Work out the finished part from the listing and answer in its coordinate system (mm). A direction names the side the tool comes from. Coordinates: 2 decimals unless noted, no trailing zeros. Loops run counter-clockwise (first coordinate to the right, second up) from the corner with the lowest first, then second, coordinate; pieces in that order, holes last.
```python
from build123d import *

# Parameters (mm, degrees)
SKETCH1_R                = 12.7
SKETCH1_R_2              = 10.9
BOSS_EXTRUDE1_DEPTH      = 71
BOSS_EXTRUDE2_DEPTH      = 63
CUT_EXTRUDE1_DEPTH       = 8
CUT_EXTRUDE2_DEPTH       = 15
CUT_EXTRUDE2_DEPTH_BACK  = 16
SKETCH4_R                = 22.297733005
SKETCH5_R                = 2
CUT_EXTRUDE3_DEPTH       = 4
CUT_EXTRUDE4_START       = -4
SKETCH6_R                = 2
CUT_EXTRUDE4_DEPTH       = 4
BOSS_EXTRUDE3_DEPTH      = 6.5
BOSS_EXTRUDE3_DEPTH_BACK = 6.5
SKETCH15_R               = 4
CUT_EXTRUDE14_DEPTH      = 7.5
BOSS_EXTRUDE4_START      = 1.75
SKETCH16_W               = 13
SKETCH16_H               = 13
SKETCH16_R               = 4
BOSS_EXTRUDE4_DEPTH      = 1.75
FILLET1_R                = 2.38
FILLET2_R                = 2.38


with BuildPart() as part:
    # Sketch1 → Boss-Extrude1 (new body)
    with BuildSketch(Plane(origin=(0, 0, 0), x_dir=(1, 0, 0), z_dir=(0, 1, 0))):
        with Locations(Location((0, 0, 0), (0, 0, 270))):
            Circle(SKETCH1_R)
        with Locations(Location((0, 0, 0), (0, 0, 270))):
            Circle(SKETCH1_R_2, mode=Mode.SUBTRACT)
    extrude(amount=BOSS_EXTRUDE1_DEPTH)

    # Sketch2 → Boss-Extrude2 (add)
    with BuildSketch(Plane.XZ):
        with BuildLine():
            Line((12.7, 12.7), (0, 12.7))
            ThreePointArc((0, 12.7), (8.980256121, 8.980256121), (12.7, 0))
            Line((12.7, 0), (12.7, 12.7))
        make_face()
        with BuildLine():
            Line((12.7, -12.7), (12.7, 0))
            ThreePointArc((12.7, 0), (8.980256121, -8.980256121), (0, -12.7))
            Line((0, -12.7), (12.7, -12.7))
        make_face()
    extrude(amount=-BOSS_EXTRUDE2_DEPTH)

    # Sketch3 → Cut-Extrude1 (cut)
    with BuildSketch(Plane.XZ):
        with BuildLine():
            Line((12.7, 12.7), (0, 12.7))
            ThreePointArc((0, 12.7), (8.980256109, 8.980256133), (12.7, 3.4e-08))
            Line((12.7, 3.4e-08), (12.7, 12.7))
        make_face()
        with BuildLine():
            Line((12.7, -12.7), (12.7, 3.4e-08))
            ThreePointArc((12.7, 3.4e-08), (8.980256133, -8.980256109), (0, -12.7))
            Line((0, -12.7), (12.7, -12.7))
        make_face()
    extrude(amount=-CUT_EXTRUDE1_DEPTH, mode=Mode.SUBTRACT)

    # Sketch4 → Cut-Extrude2 (cut, two sides: drawn at the far end of the back side and taken through both)
    with BuildSketch(Plane.XY.offset(-CUT_EXTRUDE2_DEPTH_BACK)):
        with Locations((22.331187996, 35.5)):
            Circle(SKETCH4_R)
    extrude(amount=CUT_EXTRUDE2_DEPTH + CUT_EXTRUDE2_DEPTH_BACK, mode=Mode.SUBTRACT)

    # Sketch5 → Cut-Extrude3 (cut)
    with BuildSketch(Plane(origin=(0, 0, -12.7), x_dir=(-1, 0, 0), z_dir=(0, 0, -1))):
        with Locations((-8.7, 58.5)):
            Circle(SKETCH5_R)
        with Locations((-8.7, 12.5)):
            Circle(SKETCH5_R)
    extrude(amount=-CUT_EXTRUDE3_DEPTH, mode=Mode.SUBTRACT)

    # Sketch6 → Cut-Extrude4 (cut)
    with BuildSketch(Plane.XY.offset(12.7).offset(CUT_EXTRUDE4_START)):
        with Locations(Location((8.7, 58.5, 0), (0, 0, 180))):
            Circle(SKETCH6_R)
        with Locations(Location((8.7, 12.5, 0), (0, 0, 180))):
            Circle(SKETCH6_R)
    extrude(amount=CUT_EXTRUDE4_DEPTH, mode=Mode.SUBTRACT)

    # Sketch14 → Boss-Extrude3 (add, two sides: drawn at the far end of the back side and taken through both)
    with BuildSketch(Plane(origin=(0, 35.5, 0), x_dir=(1, 0, 0), z_dir=(0, 1, 0)).offset(-BOSS_EXTRUDE3_DEPTH_BACK)):
        with BuildLine():
            Line((-14.4365, -6.5), (-14.4365, 6.5))
            Line((-14.4365, 6.5), (-10.836564596, 6.5))
            ThreePointArc((-10.836564596, 6.5), (-12.6365, 0), (-10.836564596, -6.5))
            Line((-10.836564596, -6.5), (-14.4365, -6.5))
        make_face()
    extrude(amount=BOSS_EXTRUDE3_DEPTH + BOSS_EXTRUDE3_DEPTH_BACK)

    # Sketch15 → Cut-Extrude14 (cut)
    with BuildSketch(Plane.ZY.offset(14.4365)):
        with Locations((0, 35.5)):
            Circle(SKETCH15_R)
    extrude(amount=-CUT_EXTRUDE14_DEPTH, mode=Mode.SUBTRACT)

    # Sketch16 → Boss-Extrude4 (add)
    with BuildSketch(Plane.ZY.offset(14.4365).offset(BOSS_EXTRUDE4_START)):
        with Locations((0, 35.5)):
            Rectangle(SKETCH16_W, SKETCH16_H)
        with Locations((0, 35.5)):
            Circle(SKETCH16_R, mode=Mode.SUBTRACT)
    extrude(amount=-BOSS_EXTRUDE4_DEPTH)

    # Fillet1
    fillet1_edges = [part.edges().sort_by_distance(p)[0] for p in [
        (-13.548522679, 29, 6.5),
        (-13.548522679, 29, -6.5),
        (-13.548522679, 42, -6.5),
        (-13.548522679, 42, 6.5),
    ]]
    fillet(fillet1_edges, radius=FILLET1_R)

    # Fillet2
    fillet2_edges = [part.edges().sort_by_distance(p)[0] for p in [
        (12.7, 15.389576958, 0),
        (12.7, 55.610423042, 0),
    ]]
    fillet(fillet2_edges, radius=FILLET2_R)


solid = part.part
```
1. A cutting plane is placed at B-B, the plane x = 5. Give the vertices of the cut face in (y, z).
2. Straight lines are drawn through the part: probe 1 along Y at (x, z) = (8.7, 11.5); probe 2 along X at (y, z) = (58.5, 9.85); probe 3 along Z at (x, y) = (-0.5, 3). For each, find the intervals that lie inside material, in ascending order.
3. A cutting plane is placed at A-A, the plane z = 9.75. Give the vertices of the cut face in (x, y).
4. Each of these flat-tipped pins is pushed along its axis until it touches: P1, Ø1.6, axis at x = -14, y = 36, coming from the +Z side; P2, Ø13, axis at y = 35.5, z = 0, coming from the +X side; P3, Ø4, axis at y = 26, z = -7, coming from the +X side; P4, Ø6.5, axis at x = 4.5, z = -4.5, coming from the -Y side. Where does it stop, or does it pass through?
5. For faces 4 (the cylindrical face through (-13.585, 29.716, -5.821)), 5 (the flat face through (10, 63, -10)), 6 (the cylindrical face through (7.625, 14.186, -10.728)), 7 (the flat face through (9, 12, 8.7)), determine the directions among +Z, -Z, +X, -X, +Y, -Y from which every point of the face is accessible in a straight line to the end or side of a thin tool.
6. A cutting plane is placed at D-D, the plane z = -0.75. Count the separate pieces of the cut face and the enclosed holes in it, then the cut area to 3 significant figures.
7. Determine the mould class of faces 1 (the cylindrical face through (-13.205, 35.676, -3.996)), 2 (the flat face through (0.6, 29, -12.7)), 3 (the flat face through (12.7, 11, 0)) for opening direction Z: released by +Z, released by -Z, zero draft, split by the parting line, or undercut.
8. A cutting plane is placed at C-C, the plane y = 12.5. Give the vertices of the cut face in (x, z), then the cut area to 3 significant figures.
Answers below:
1. outline: (0, -11.67) - (8, -11.67) - (8, -12.7) - (21.47, -12.7) - (21.47, -9.69) - (0, -9.69) - close; (0, 9.69) - (21.47, 9.69) - (21.47, 12.7) - (8, 12.7) - (8, 11.67) - (0, 11.67) - close; (49.53, -12.7) - (63, -12.7) - (63, -11.67) - (71, -11.67) - (71, -9.69) - (49.53, -9.69) - close; (49.53, 9.69) - (71, 9.69) - (71, 11.67) - (63, 11.67) - (63, 12.7) - (49.53, 12.7) - close
2. probe 1: y = 8 to 10.5, 14.5 to 17.85, 53.15 to 56.5, 60.5 to 63
2. probe 2: x = -8.02 to -4.67, 4.67 to 6.7, 10.7 to 12.7
2. probe 3: z = -12.69 to -10.89, 10.89 to 12.69
3. outline: (-8.14, 0) - (-4.87, 0) - (-4.87, 71) - (-8.14, 71) - close; (4.87, 0) - (8.14, 0) - (8.14, 8) - (12.7, 8) - (12.7, 13.94) arc R2.38 ccw to (11.48, 16.02) arc R22.3 cw to (4.87, 21.63) - close; (4.87, 49.37) arc R22.3 cw to (11.48, 54.98) arc R2.38 ccw to (12.7, 57.06) - (12.7, 63) - (8.14, 63) - (8.14, 71) - (4.87, 71) - close; hole circle Ø4 at (8.7, 12.5); hole circle Ø4 at (8.7, 58.5)
4. P1: stops at z = 6.5
4. P2: stops at x = -8.75
4. P3: stops at x = -6.15
4. P4: passes through
5. face 4: -Z, -X, -Y
5. face 5: -Z, +X, +Y
5. face 6: -Z
5. face 7: +Z
6. separate pieces: 4
6. enclosed holes: 0
6. area: 189 mm2
7. face 1: undercut
7. face 2: released by -Z
7. face 3: zero draft
8. outline: (0, -12.7) - (6.7, -12.7) - (6.7, -8.7) - (10.7, -8.7) - (10.7, -12.7) - (12.7, -12.7) - (12.7, 12.7) - (10.7, 12.7) - (10.7, 8.7) - (6.7, 8.7) - (6.7, 12.7) - (0, 12.7) arc R12.7 ccw to start; hole circle Ø21.8 at (0, 0)
8. area: 171 mm2
